Design review of the part built by this model. Coordinates are the model's own, in mm. A direction names the side the tool comes from. Coordinates: 2 decimals unless noted, no trailing zeros. Loops run counter-clockwise (first coordinate to the right, second up) from the corner with the lowest first, then second, coordinate; pieces in that order, holes last. Notation, with made-up numbers: M -15.5,46.5 L 6.5,46.5 A16 ccw 6.5,66.5 Z; hole C 58,18 d3. An arc over 180 degrees is marked long. Answer as a JSON object with one key per item and string values. Group by question number.
1. To check wall thickness, follow probe 1 along X at (y, z) = (-65, 3.45); probe 2 along Y at (x, z) = (18.5, 2.25); probe 3 along Y at (x, z) = (71, 4.45). State the ranges of each line that lie inside material, in increasing order.
2. Consider section B-B (x = 5.5). State the section outline as (y, z) points, then the cut area to 3 significant figures.
3. Draft analysis for pull direction X (two halves, no side actions). For faces 3 (the flat face through (149.585, -120.909, 3.621)), 4 (the flat face through (64, -100, 2.1)), 5 (the flat face through (142.35, -117.44, 3.62)), 6 (the flat face through (146.971, -98.467, 3.621)), state which applies: +X half, -X half, draft (parallel to the pull), parting line (faces both ways), or undercut.
4. Consider section A-A (y = -10). State the section outline as (x, z) points, then the cut area to 3 significant figures.
5. Insertion check: pin 1 (0.9 mm diameter, centred on x = 44, z = 4, fed in from -Y); pin 2 (0.7 mm diameter, centred on y = -111.5, z = 4, fed in from +X); pin 3 (1.5 mm diameter, centred on x = 116, z = 4, fed in from -Y). Each pin has a flat end and moves straight along its axis. Give the tip position at first contact, or say it passes through.
6. Machinability: for faces 1 (the flat face through (156.46, -94.71, 3.62)), 2 (the flat face through (103.01, -115.79, 3.62)), which of the approach directions +Z, -Z, +X, -X, +Y, -Y give a long, thin tool a straight path to every point of the face, cutting with its end or side? Answer none if there is none.
Solid Edge part; units mm, degrees
sketch "Sketch1" plane through (74.3033, -64.1291, 5.1) normal (0, 0, 1) x (1, 0, 0)
  line L0 (-45.2193, 73.1597) -> (-28.1693, 73.1597)
  arc A0 (-28.1693, 73.1597) -> (-27.1693, 74.1597) centre (-28.1693, 74.1597) ccw
  line L1 (-27.1693, 74.1597) -> (-27.1693, 75.0138)
  arc A1 (-26.1693, 76.0138) -> (-27.1693, 75.0138) centre (-26.1693, 75.0138) ccw
  line L2 (-26.1693, 76.0138) -> (10.8807, 76.0138)
  arc A2 (10.8807, 76.0138) -> (11.8807, 75.0138) centre (10.8807, 75.0138) cw
  line L3 (11.8807, 75.0138) -> (11.8807, 74.1563)
  arc A3 (12.8807, 73.1563) -> (11.8807, 74.1563) centre (12.8807, 74.1563) cw
  line L4 (12.8807, 73.1563) -> (29.9307, 73.1563)
  arc A4 (29.9307, 73.1563) -> (30.9307, 72.1563) centre (29.9307, 72.1563) cw
  line L5 (30.9307, 72.1563) -> (30.9307, 71.2986)
  arc A5 (31.9307, 70.2986) -> (30.9307, 71.2986) centre (31.9307, 71.2986) cw
  line L6 (31.9307, 70.2986) -> (75.1733, 70.2986)
  arc A6 (75.1733, 70.2986) -> (76.1733, 69.2986) centre (75.1733, 69.2986) cw
  line L7 (76.1733, 69.2986) -> (76.1733, -26.5472)
  arc A7 (76.1733, -26.5472) -> (76.6733, -27.4132) centre (77.1733, -26.5472) ccw
  line L8 (87.48, -33.6525) -> (76.6733, -27.4132)
  arc A8 (87.48, -33.6525) -> (87.8461, -35.0185) centre (86.98, -34.5185) cw
  line L9 (87.8461, -35.0185) -> (62.3613, -79.1594)
  arc A9 (60.9953, -79.5254) -> (62.3613, -79.1594) centre (61.4953, -78.6594) ccw
  line L10 (-1.9566, -43.1802) -> (60.9953, -79.5254)
  arc A10 (-2.4566, -43.0462) -> (-1.9566, -43.1802) centre (-2.4566, -44.0462) cw
  line L11 (-6.1693, -43.0462) -> (-2.4566, -43.0462)
  arc A11 (-6.1693, -43.0462) -> (-7.1693, -44.0462) centre (-6.1693, -44.0462) ccw
  line L12 (-7.1693, -44.9037) -> (-7.1693, -44.0462)
  arc A12 (-8.1693, -45.9037) -> (-7.1693, -44.9037) centre (-8.1693, -44.9037) ccw
  line L13 (-25.2193, -45.9037) -> (-8.1693, -45.9037)
  arc A13 (-26.2193, -46.9037) -> (-25.2193, -45.9037) centre (-25.2193, -46.9037) cw
  line L14 (-26.2193, -47.7612) -> (-26.2193, -46.9037)
  arc A14 (-27.2193, -48.7612) -> (-26.2193, -47.7612) centre (-27.2193, -47.7612) ccw
  line L15 (-83.3193, -48.7612) -> (-27.2193, -48.7612)
  arc A15 (-84.3193, -47.7612) -> (-83.3193, -48.7612) centre (-83.3193, -47.7612) ccw
  line L16 (-84.3193, 69.2988) -> (-84.3193, -47.7612)
  arc A16 (-84.3193, 69.2988) -> (-83.3193, 70.2988) centre (-83.3193, 69.2988) cw
  line L17 (-83.3193, 70.2988) -> (-47.2193, 70.2988)
  arc A17 (-47.2193, 70.2988) -> (-46.2193, 71.2988) centre (-47.2193, 71.2988) ccw
  line L18 (-46.2193, 71.2988) -> (-46.2193, 72.1597)
  arc A18 (-46.2193, 72.1597) -> (-45.2193, 73.1597) centre (-45.2193, 72.1597) cw
  line L19 (-18.1693, 68.0138) -> (2.8807, 68.0138)
  arc A19 (2.8807, 68.0138) -> (3.8807, 67.0138) centre (2.8807, 67.0138) cw
  line L20 (3.8807, 67.0138) -> (3.8807, 66.1563)
  arc A20 (4.8807, 65.1563) -> (3.8807, 66.1563) centre (4.8807, 66.1563) cw
  line L21 (4.8807, 65.1563) -> (21.9307, 65.1563)
  arc A21 (21.9307, 65.1563) -> (22.9307, 64.1563) centre (21.9307, 64.1563) cw
  line L22 (22.9307, 64.1563) -> (22.9307, 63.2986)
  arc A22 (23.9307, 62.2986) -> (22.9307, 63.2986) centre (23.9307, 63.2986) cw
  line L23 (23.9307, 62.2986) -> (67.1733, 62.2986)
  arc A23 (67.1733, 62.2986) -> (68.1733, 61.2986) centre (67.1733, 61.2986) cw
  line L24 (68.1733, 61.2986) -> (68.1733, -31.1662)
  arc A24 (68.1733, -31.1662) -> (68.6733, -32.0322) centre (69.1733, -31.1662) ccw
  line L25 (76.5517, -36.5808) -> (68.6733, -32.0322)
  arc A25 (76.5517, -36.5808) -> (76.9178, -37.9468) centre (76.0517, -37.4468) cw
  line L26 (59.4268, -68.2421) -> (76.9178, -37.9468)
  arc A26 (58.0608, -68.6081) -> (59.4268, -68.2421) centre (58.5608, -67.7421) ccw
  line L27 (0.1618, -35.1802) -> (58.0608, -68.6081)
  arc A27 (-0.3382, -35.0462) -> (0.1618, -35.1802) centre (-0.3382, -36.0462) cw
  line L28 (-14.1693, -35.0462) -> (-0.3382, -35.0462)
  arc A28 (-14.1693, -35.0462) -> (-15.1693, -36.0462) centre (-14.1693, -36.0462) ccw
  line L29 (-15.1693, -36.9037) -> (-15.1693, -36.0462)
  arc A29 (-16.1693, -37.9037) -> (-15.1693, -36.9037) centre (-16.1693, -36.9037) ccw
  line L30 (-33.2193, -37.9037) -> (-16.1693, -37.9037)
  arc A30 (-34.2193, -38.9037) -> (-33.2193, -37.9037) centre (-33.2193, -38.9037) cw
  line L31 (-34.2193, -39.7612) -> (-34.2193, -38.9037)
  arc A31 (-35.2193, -40.7612) -> (-34.2193, -39.7612) centre (-35.2193, -39.7612) ccw
  line L32 (-75.3193, -40.7612) -> (-35.2193, -40.7612)
  arc A32 (-76.3193, -39.7612) -> (-75.3193, -40.7612) centre (-75.3193, -39.7612) ccw
  line L33 (-76.3193, 61.2988) -> (-76.3193, -39.7612)
  arc A33 (-76.3193, 61.2988) -> (-75.3193, 62.2988) centre (-75.3193, 61.2988) cw
  line L34 (-75.3193, 62.2988) -> (-39.2193, 62.2988)
  arc A34 (-39.2193, 62.2988) -> (-38.2193, 63.2988) centre (-39.2193, 63.2988) ccw
  line L35 (-38.2193, 63.2988) -> (-38.2193, 64.1597)
  arc A35 (-38.2193, 64.1597) -> (-37.2193, 65.1597) centre (-37.2193, 64.1597) cw
  line L36 (-37.2193, 65.1597) -> (-20.1693, 65.1597)
  arc A36 (-20.1693, 65.1597) -> (-19.1693, 66.1597) centre (-20.1693, 66.1597) ccw
  line L37 (-19.1693, 66.1597) -> (-19.1693, 67.0138)
  arc A37 (-18.1693, 68.0138) -> (-19.1693, 67.0138) centre (-18.1693, 67.0138) ccw
extrude "ExtrudedProtrusion_4" add sketch "Sketch1" against normal blind 3
properties material "ABS Plastic, high impact"
Findings below:
{
 "1": {"probe 1": "x = -10.02 to -2.02, 142.48 to 150.48", "probe 2": "y = -112.89 to -104.89, -1.83 to 6.17", "probe 3": "y = -107.18 to -99.18, 3.88 to 11.88"},
 "2": {"outline": "M -112.89,2.1 L -104.89,2.1 L -104.89,5.1 L -112.89,5.1 Z; M -1.83,2.1 L 6.17,2.1 L 6.17,5.1 L -1.83,5.1 Z", "area": "48.0 mm^2"},
 "3": {"face 3": "+X half", "face 4": "draft", "face 5": "undercut", "face 6": "undercut"},
 "4": {"outline": "M -10.02,2.1 L -2.02,2.1 L -2.02,5.1 L -10.02,5.1 Z; M 142.48,2.1 L 150.48,2.1 L 150.48,5.1 L 142.48,5.1 Z", "area": "48.0 mm^2"},
 "5": {"pin 1": "stops at y = -112.89", "pin 2": "stops at x = 155.22", "pin 3": "stops at y = -132.95"},
 "6": {"face 1": "+Z, -Z, +X, +Y", "face 2": "+Z, -Z"}
}
